```python
from build123d import *

# Parameters (mm, degrees)
EXTRUDE_1_DEPTH     = 12
SKETCH_2_R          = 6.75
CUT_EXTRUDE_1_DEPTH = 8.5
SKETCH_4_R          = 7
EXTRUDE_2_DEPTH     = 3
SKETCH_3_R          = 3.4
CUT_EXTRUDE_2_DEPTH = 33.74522866
CHAMFER_1_SIZE      = 0.2


with BuildPart() as part:
    # 草图1 → 凸台-拉伸1 (new body)
    with BuildSketch(Plane(origin=(0, 0, 0), x_dir=(1, 0, 0), z_dir=(0, 1, 0))):
        with BuildLine():
            Line((-5, -28), (-5, -8.660254038))
            ThreePointArc((-5, -8.660254038), (-10, 0), (-5, 8.660254038))
            Line((-5, 8.660254038), (-5, 28))
            ThreePointArc((-5, 28), (-4.414213562, 29.414213562), (-3, 30))
            Line((-3, 30), (3, 30))
            ThreePointArc((3, 30), (4.414213562, 29.414213562), (5, 28))
            Line((5, 28), (5, 8.660254038))
            ThreePointArc((5, 8.660254038), (10, 0), (5, -8.660254038))
            Line((5, -8.660254038), (5, -28))
            ThreePointArc((5, -28), (4.414213562, -29.414213562), (3, -30))
            Line((3, -30), (-3, -30))
            ThreePointArc((-3, -30), (-4.414213562, -29.414213562), (-5, -28))
        make_face()
    extrude(amount=EXTRUDE_1_DEPTH)

    # 草图2 → 切除-拉伸1 (cut)
    with BuildSketch(Plane.XZ):
        with Locations(Location((0, 0, 0), (0, 0, 270))):
            Circle(SKETCH_2_R)
    extrude(amount=-CUT_EXTRUDE_1_DEPTH, mode=Mode.SUBTRACT)

    # 草图4 → 凸台-拉伸2 (add)
    with BuildSketch(Plane(origin=(0, 12, 0), x_dir=(1, 0, 0), z_dir=(0, 1, 0))):
        with Locations(Location((0, 0, 0), (0, 0, 270))):
            Circle(SKETCH_4_R)
    extrude(amount=EXTRUDE_2_DEPTH)

    # 草图3 → 切除-拉伸2 (cut, through all)
    with BuildSketch(Plane.XZ.offset(-8.5)):
        with Locations(Location((0, 0, 0), (0, 0, 270))):
            Circle(SKETCH_3_R)
    extrude(amount=-CUT_EXTRUDE_2_DEPTH, mode=Mode.SUBTRACT)

    # 倒角1
    chamfer_1_edges = [part.edges().sort_by_distance(p)[0] for p in [
        (5, 0, 18.330127019),
        (4.414213562, 0, 29.414213562),
        (4.414213562, 12, -29.414213562),
        (0, 0, 30),
        (-4.414213562, 0, 29.414213562),
        (-5, 0, 18.330127019),
        (-10, 0, 0),
        (-5, 0, -18.330127019),
        (-4.414213562, 0, -29.414213562),
        (0, 0, -30),
        (4.414213562, 0, -29.414213562),
        (5, 0, -18.330127019),
        (10, 0, 0),
        (0, 12, -30),
        (-4.414213562, 12, -29.414213562),
        (-5, 12, -18.330127019),
        (-10, 12, 0),
        (-5, 12, 18.330127019),
        (-4.414213562, 12, 29.414213562),
        (0, 0, 6.75),
        (0, 12, 30),
        (0, 15, -7),
        (4.414213562, 12, 29.414213562),
        (0, 15, 3.4),
        (5, 12, 18.330127019),
        (10, 12, 0),
        (5, 12, -18.330127019),
    ]]
    chamfer(chamfer_1_edges, length=CHAMFER_1_SIZE)


solid = part.part
```
Part model, mm, in its own coordinate system. A direction names the side the tool comes from. Coordinates: 2 decimals unless noted, no trailing zeros. Order: outer loops, then holes, each group sorted by start corner. A loop starts at its lowest first (then second) coordinate and runs counter-clockwise, first axis right, second up. Notation, with made-up numbers: (44.5, -37) - (103.5, -37) arc R18 cw to (103.5, -3) - close; hole circle Ø9 at (28.25, 8.25). An arc over 180 degrees is marked (long way). Return JSON: item names as keys, results as strings. Group by question number.
Item 1: Pin check, flat tips, straight feed: pin 1 (11 mm diameter, centred on x = 0, z = 0, fed in from +Y); pin 2 (6 mm diameter, centred on y = 6, z = 18, fed in from -X); pin 3 (4 mm diameter, centred on y = 5, z = 7, fed in from -X); pin 4 (1.5 mm diameter, centred on x = -7, y = 5.5, fed in from -Z). Stop position of each tip, or through.
Item 2: Which spindle directions (+Z, -Z, +X, -X, +Y, -Y) get a long thin tool onto all of the face, cutting with end or side? Do faces 1 (the face through (-6.834, 13.38, -1.517)), 2 (the face through (-5, 6, -18)), 3 (the face through (-3.32, 11.61, 0.74)), 4 (the face through (-6.59, 4.29, 1.46)). Say none if no direction does.
Item 3: Drill centre lines: probe 1 along X at (y, z) = (11, -20); probe 2 along Y at (x, z) = (2.25, 12); probe 3 along Z at (x, y) = (2.5, 3.75). Where is each one in solid material? Low to high. Write a range as from..to.
Item 4: Cut at D-D (z = 16.5). List the corners of the cut face in (x, y).
Item 5: Pull direction X, two halves, no side cores. Call faces 5 (the face through (-4.4, 5.92, 29.43)), 6 (the face through (5, 6, 18)), 7 (the face through (3, 8.5, 2)): pulls with the +X half, pulls with the -X half, needs draft (parallel to the pull), parting line crosses it, or undercut.
Item 6: Cut at A-A (x = 0). List the corners of the cut face in (y, z).
Item 7: Cut at C-C (z = 0). List the corners of the cut face in (x, y), plus the area to 3 significant figures.
Item 8: Cut at B-B (y = 10.5). List the corners of the cut face in (x, z), plus the area to 3 significant figures.
Check values:
{
 "1": {"pin 1": "stops at y = 15", "pin 2": "stops at x = -5", "pin 3": "stops at x = -8.66", "pin 4": "stops at z = -7.81"},
 "2": {"face 1": "+Y", "face 2": "-Z, -X, +Y, -Y", "face 3": "+Y, -Y", "face 4": "-Y"},
 "3": {"probe 1": "x = -5..5", "probe 2": "y = 0..12", "probe 3": "z = -30..-6.27, 6.27..30"},
 "4": {"outline": "(-5, 0.2) - (-4.8, 0) - (4.8, 0) - (5, 0.2) - (5, 11.8) - (4.8, 12) - (-4.8, 12) - (-5, 11.8) - close"},
 "5": {"face 5": "pulls with the -X half", "face 6": "pulls with the +X half", "face 7": "undercut"},
 "6": {"outline": "(0, -29.8) - (0.2, -30) - (11.8, -30) - (12, -29.8) - (12, -7) - (14.8, -7) - (15, -6.8) - (15, -3.6) - (14.8, -3.4) - (8.5, -3.4) - (8.5, -6.75) - (0.2, -6.75) - (0, -6.95) - close; (0, 6.95) - (0.2, 6.75) - (8.5, 6.75) - (8.5, 3.4) - (14.8, 3.4) - (15, 3.6) - (15, 6.8) - (14.8, 7) - (12, 7) - (12, 29.8) - (11.8, 30) - (0.2, 30) - (0, 29.8) - close"},
 "7": {"outline": "(-10, 0.2) - (-9.8, 0) - (-6.95, 0) - (-6.75, 0.2) - (-6.75, 8.5) - (-3.4, 8.5) - (-3.4, 14.8) - (-3.6, 15) - (-6.8, 15) - (-7, 14.8) - (-7, 12) - (-9.8, 12) - (-10, 11.8) - close; (3.4, 8.5) - (6.75, 8.5) - (6.75, 0.2) - (6.95, 0) - (9.8, 0) - (10, 0.2) - (10, 11.8) - (9.8, 12) - (7, 12) - (7, 14.8) - (6.8, 15) - (3.6, 15) - (3.4, 14.8) - close", "area": "123 mm2"},
 "8": {"outline": "(-5, -28) arc R2 ccw to (-3, -30) - (3, -30) arc R2 ccw to (5, -28) - (5, -8.66) arc R10 ccw to (5, 8.66) - (5, 28) arc R2 ccw to (3, 30) - (-3, 30) arc R2 ccw to (-5, 28) - (-5, 8.66) arc R10 ccw to (-5, -8.66) - close; hole circle Ø6.8 at (0, 0)", "area": "683 mm2"}
}
